Design review of the part built by this model. Coordinates are the model's own, in mm. A direction names the side the tool comes from. Coordinates: 2 decimals unless noted, no trailing zeros. Loops run counter-clockwise (first coordinate to the right, second up) from the corner with the lowest first, then second, coordinate; pieces in that order, holes last. Notation, with made-up numbers: (-25.75, 41.25) -> (11.25, 41.25) arc R33 cw to (11.25, 69.25) -> close; hole circle Ø4 at (44, -10.5). An arc over 180 degrees is marked (long way). Answer as a JSON object with one key per item and string values.
```python
from build123d import *
from OCP.BRepFilletAPI import BRepFilletAPI_MakeChamfer

# Parameters (mm, degrees)
SKETCH1_W           = 15
SKETCH1_H           = 12
BOSS_EXTRUDE1_DEPTH = 6
SKETCH1_3_W         = 15
SKETCH1_3_H         = 26
SKETCH1_3_R         = 1.7
BOSS_EXTRUDE2_DEPTH = 3
CHAMFER1_SIZE       = 3
CUT_EXTRUDE1_DEPTH  = 6
CHAMFER2_SIZE       = 2.5
CHAMFER2_SIZE2      = 2.451963608


with BuildPart() as part:
    # Sketch1 → Boss-Extrude1 (new body)
    with BuildSketch(Plane(origin=(0, 0, 0), x_dir=(-1, 0, 0), z_dir=(0, 1, 0))):
        with BuildLine():
            Line((-7.5, -8), (-15, -8))
            Line((-15, -8), (-15, -20))
            Line((-15, -20), (-7.5, -20))
            Line((-7.5, -20), (-7.5, -16.05121915))
            ThreePointArc((-7.5, -16.05121915), (-10.05, -14), (-7.5, -11.94878085))
            Line((-7.5, -11.94878085), (-7.5, -8))
        make_face()
        with BuildLine():
            Line((7.5, -8), (-7.5, -8))
            Line((-7.5, -8), (-7.5, -11.94878085))
            ThreePointArc((-7.5, -11.94878085), (-6.313693183, -12.683755342), (-5.85, -14))
            ThreePointArc((-5.85, -14), (-6.313693183, -15.316244658), (-7.5, -16.05121915))
            Line((-7.5, -16.05121915), (-7.5, -20))
            Line((-7.5, -20), (7.5, -20))
            Line((7.5, -20), (7.5, -16.05121915))
            ThreePointArc((7.5, -16.05121915), (5.85, -14), (7.5, -11.94878085))
            Line((7.5, -11.94878085), (7.5, -8))
        make_face()
        with BuildLine():
            Line((15, -8), (7.5, -8))
            Line((7.5, -8), (7.5, -11.94878085))
            ThreePointArc((7.5, -11.94878085), (9.266244658, -12.363693183), (10.05, -14))
            ThreePointArc((10.05, -14), (9.266244658, -15.636306817), (7.5, -16.05121915))
            Line((7.5, -16.05121915), (7.5, -20))
            Line((7.5, -20), (15, -20))
            Line((15, -20), (15, -8))
        make_face()
        Polygon((15, -8), (7.5, 4), (7.5, -8), align=None)
        with Locations((0, -2)):
            Rectangle(SKETCH1_W, SKETCH1_H)
        Polygon((-7.5, 4), (-15, -8), (-7.5, -8), align=None)
    extrude(amount=BOSS_EXTRUDE1_DEPTH)

    # Sketch1<3> → Boss-Extrude2 (add)
    with BuildSketch(Plane(origin=(0, 0, 0), x_dir=(-1, 0, 0), z_dir=(0, 1, 0))):
        with Locations((0, 17)):
            Rectangle(SKETCH1_3_W, SKETCH1_3_H)
        with Locations(Location((0, 25.8, 0), (0, 0, 90))):
            Circle(SKETCH1_3_R, mode=Mode.SUBTRACT)
    extrude(amount=BOSS_EXTRUDE2_DEPTH)

    # Chamfer1
    chamfer1_edges = [part.edges().sort_by_distance(p)[0] for p in [
        (0, 3, 4),
    ]]
    chamfer(chamfer1_edges, length=CHAMFER1_SIZE - 0.0001)  # a hair under: the kernel refuses the full size

    # Sketch2 → Cut-Extrude1 (cut)
    with BuildSketch(Plane(origin=(0, 6, 0), x_dir=(-1, 0, 0), z_dir=(0, 1, 0))):
        Polygon((-5.837257075, 1), (-11.462257075, -8), (11.462257075, -8), (5.837257075, 1), align=None)
    extrude(amount=-CUT_EXTRUDE1_DEPTH, mode=Mode.SUBTRACT)

    # Chamfer2: one chamfer whose edges measure the first distance from different faces: ONE call of the kernel's chamfer builder (chamfer() names one face for all edges)
    chamfer2_edges_1 = [part.edges().sort_by_distance(p)[0] for p in [
        (-11.462257075, 3, -8),
    ]]
    chamfer2_side_1 = [part.faces().sort_by_distance(p)[0] for p in [
        (0, 3, -8),
    ]]
    chamfer2_edges_2 = [part.edges().sort_by_distance(p)[0] for p in [
        (11.462257075, 3, -8),
    ]]
    chamfer2_side_2 = [part.faces().sort_by_distance(p)[0] for p in [
        (8.649757075, 3, -3.5),
    ]]
    chamfer2 = BRepFilletAPI_MakeChamfer(part.part.solid().wrapped)
    for e in chamfer2_edges_1:
        chamfer2.Add(CHAMFER2_SIZE, CHAMFER2_SIZE2, e.wrapped, chamfer2_side_1[0].wrapped)  # the first distance lies on this face
    for e in chamfer2_edges_2:
        chamfer2.Add(CHAMFER2_SIZE, CHAMFER2_SIZE2, e.wrapped, chamfer2_side_2[0].wrapped)  # the first distance lies on this face
    add(Compound.cast(chamfer2.Shape()), mode=Mode.REPLACE)


solid = part.part
```
1) Add section A-A, the plane z = 25.8. Give the boundary of the cut face in (x, y), and give its area (3 significant figures).
Completed:
{"outline": "(-7.5, 0) -> (-1.7, 0) -> (-1.7, 3) -> (-7.5, 3) -> close; (1.7, 0) -> (7.5, 0) -> (7.5, 3) -> (1.7, 3) -> close", "area": "34.8 mm²"}
2) Wall thickness on probe 1 along X at (y, z) = (4.2, -14); probe 2 along X at (y, z) = (2.05, 25.8); probe 3 along Z at (x, y) = (5.5, 1.75): over which ranges is each line inside the solid? List them lowest first.
Completed:
{"probe 1": "-15 to -10.05, -5.85 to 5.85, 10.05 to 15", "probe 2": "-7.5 to -1.7, 1.7 to 7.5", "probe 3": "-20 to -8, 1 to 30"}
3) Clearance check with flat-ended pins moving along their axes: pin 1 Ø2 at (y, z) = (4.5, 0.5) entering from +X; pin 2 Ø2.5 at (x, z) = (7.95, -14) entering from +Y; pin 3 Ø4 at (x, z) = (8.5, 11) entering from +Y; pin 4 Ø3 at (x, y) = (-10.5, 2.5) entering from +Z. State where each tip first meets the part, or that it passes through.
Completed:
{"pin 1": "x = 10.31", "pin 2": "through", "pin 3": "y = 3", "pin 4": "z = 1.6"}
4) The part is to be moulded in two halves that separate along Z. For faces 4 (the flat face through (0, 3, 19)), 5 (the flat face through (0, 3, 1)), 6 (the flat face through (0, 1, 30)), 7 (the flat face through (0, 3, -20)), say which applies: pulls with the +Z half, pulls with the -Z half, needs draft (parallel to the pull), parting line crosses it, or undercut.
Completed:
{"face 4": "needs draft", "face 5": "undercut", "face 6": "pulls with the +Z half", "face 7": "pulls with the -Z half"}
5) For faces 1 (the flat face through (9.57, 3.04, -6.95)), 2 (the flat face through (7.5, 2, 17)), 3 (the flat face through (-7.5, 2, 17)), list the 3-axis set-ups (+Z, -Z, +X, -X, +Y, -Y) from which the entire face can be reached by the end or side of a thin tool; tool diameter is ignored.
Completed:
{"face 1": "+Y, -Y", "face 2": "+Z, +X, +Y, -Y", "face 3": "+Z, -X, +Y, -Y"}
6) Add section D-D, the plane x = 12.5. Give the boundary of the cut face in (y, z), and give its area (3 significant figures).
Completed:
{"outline": "(0, -20) -> (6, -20) -> (6, -4) -> (0, -4) -> close", "area": "96.0 mm²"}
7) Add section C-C, the plane y = 2.5. Give the boundary of the cut face in (x, z), and give its area (3 significant figures).
Completed:
{"outline": "(-15, -20) -> (15, -20) -> (15, -8) -> (7.5, 4) -> (7.5, 30) -> (-7.5, 30) -> (-7.5, 4) -> (-15, -8) -> close; hole (-10.16, -5.92) -> (-8.96, -8) -> (9.01, -8) -> (10.14, -5.88) -> (5.84, 1) -> (-5.84, 1) -> close; hole circle Ø4.2 at (-7.95, -14); hole circle Ø3.4 at (0, 25.8); hole circle Ø4.2 at (7.95, -14)", "area": "833 mm²"}
8) Add section B-B, the plane x = 0. Count the separate pieces of the cut face and the enclosed holes in it, and give its area (3 significant figures).
Completed:
{"separate pieces": "3", "enclosed holes": "0", "area": "162 mm²"}
